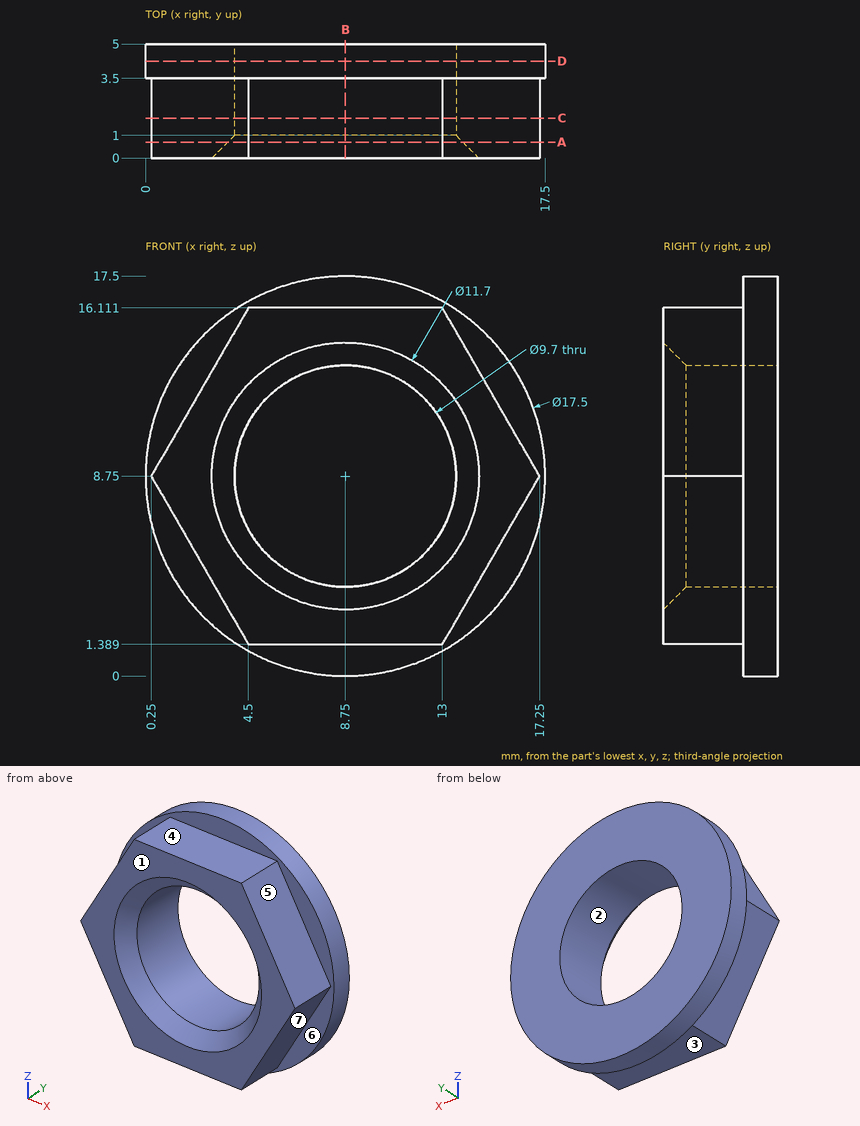
Check sheet for the drawn part. Datum: minimum x, y, z corner. Units: mm. A direction names the side the tool comes from. Coordinates: 2 decimals unless noted, no trailing zeros. Loops run counter-clockwise (first coordinate to the right, second up) from the corner with the lowest first, then second, coordinate; pieces in that order, holes last. Notation, with made-up numbers: (-1.5, 79.25) -> (40.5, 79.25) arc R23 ccw to (40.5, 118.25) -> close; hole circle Ø7 at (-35.5, -26). An arc over 180 degrees is marked (long way). Answer as a JSON object with one key per item and string values. Group by question number.
Item 1: Sectioned sample at B-B on x = 8.75. Record the boundary of the cut face in (y, z).
Item 2: Sectioned sample at D-D on y = 4.25. Record the boundary of the cut face in (x, z), plus the area to 3 significant figures.
Item 3: Tool access check on the marked faces 4, 5, 6 and 7. Record the directions out of +Z, -Z, +X, -X, +Y, -Y that give a thin tool (end or side, any length) a straight path to the whole face; none if there is none.
Item 4: Sectioned sample at C-C on y = 1.75. Record the boundary of the cut face in (x, z).
Item 5: Sectioned sample at A-A on y = 0.7. Record the boundary of the cut face in (x, z).
Item 6: Depth check by flat-ended pin: pin 1 (1.8 mm diameter, centred on x = 9, y = 2, fed in from +Z); pin 2 (2 mm diameter, centred on y = 2, z = 13, fed in from +X); pin 3 (3 mm diameter, centred on x = 6.5, y = 1, fed in from -Z). Enter the tip coordinate at first touch or a pass-through.
Item 7: Mould release check, pull along Z, two halves, no side actions. Record for the marked faces 1, 2 and 3: +Z half, -Z half, draft (parallel to the pull), parting line (faces both ways), or undercut.
Item 8: Scan lines: probe 1 along Z at (x, y) = (8.75, 2.65); probe 2 along Z at (x, y) = (8.75, 3.9); probe 3 along Y at (x, z) = (3, 15.25). Record each from-to range of solid material in increasing order.
Evaluation:
{
 "1": {"outline": "(0, 1.39) -> (3.5, 1.39) -> (3.5, 0) -> (5, 0) -> (5, 3.9) -> (1, 3.9) -> (0, 2.9) -> close; (0, 14.6) -> (1, 13.6) -> (5, 13.6) -> (5, 17.5) -> (3.5, 17.5) -> (3.5, 16.11) -> (0, 16.11) -> close"},
 "2": {"outline": "circle Ø17.5 at (8.75, 8.75); hole circle Ø9.7 at (8.75, 8.75)", "area": "167 mm²"},
 "3": {"face 4": "+Z, +X, -X, -Y", "face 5": "+Z, +X, -Y", "face 6": "-Y", "face 7": "-Z, +X, -Y"},
 "4": {"outline": "(0.25, 8.75) -> (4.5, 1.39) -> (13, 1.39) -> (17.25, 8.75) -> (13, 16.11) -> (4.5, 16.11) -> close; hole circle Ø9.7 at (8.75, 8.75)"},
 "5": {"outline": "(0.25, 8.75) -> (4.5, 1.39) -> (13, 1.39) -> (17.25, 8.75) -> (13, 16.11) -> (4.5, 16.11) -> close; hole circle Ø10.3 at (8.75, 8.75)"},
 "6": {"pin 1": "stops at z = 16.11", "pin 2": "stops at x = 15.37", "pin 3": "stops at z = 1.39"},
 "7": {"face 1": "draft", "face 2": "undercut", "face 3": "-Z half"},
 "8": {"probe 1": "z = 1.39 to 3.9, 13.6 to 16.11", "probe 2": "z = 0 to 3.9, 13.6 to 17.5", "probe 3": "y = 3.5 to 5"}
}
